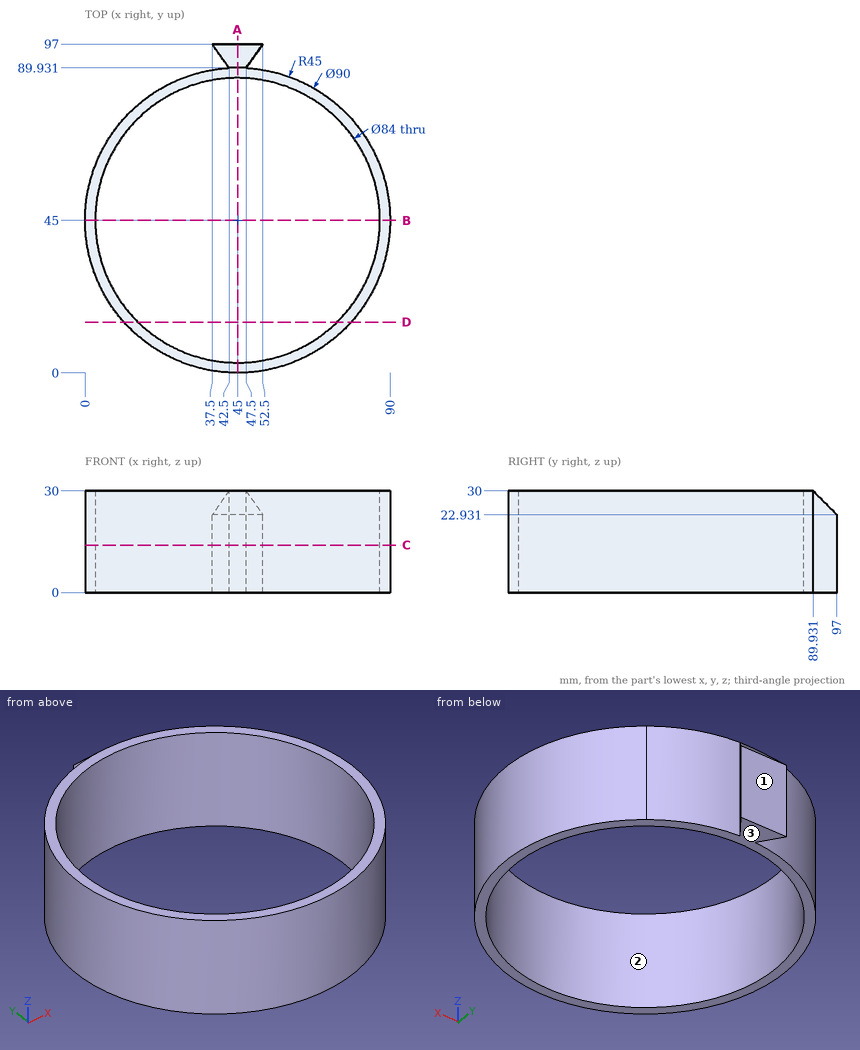
Drawing for the job (mm, zero at the part's lowest x, y, z). Round coordinates to 2 decimals unless told otherwise and drop trailing zeros. Order: outer loops, then holes, each group sorted by start corner. A loop starts at its lowest first (then second) coordinate and runs counter-clockwise, first axis right, second up. Notation, with made-up numbers: (70.25, 76) -> (124.25, 76) arc R20 ccw to (124.25, 115) -> close; hole circle Ø4 at (78, 40). An arc over 180 degrees is marked (long way). Write item = value, one per line. Start each with the question number.
(1) Pin check, flat tips, straight feed: P1, Ø12, axis at x = 11.5, z = 17, coming from the -Y side; P2, Ø2, axis at y = 38, z = 26, coming from the +X side; P3, Ø2, axis at x = 67.5, z = 26, coming from the -Y side; P4, Ø5, axis at y = 43.5, z = 12.5, coming from the -X side. Stop position of each tip, or through.
(2) Pull direction Y, two halves, no side cores. Call the marked faces 1, 2 and 3: released by +Y, released by -Y, zero draft, split by the parting line, or undercut.
(3) Cut at C-C, the plane z = 14. List the corners of the cut face in (x, y) (1 decimal).
(4) Cut at A-A, the plane x = 45. List the corners of the cut face in (y, z).
(5) Probe line 1 (Y direction, x = 45, z = 11.25); line 2 (Y direction, x = 59, z = 6.5); line 3 (X direction, y = 32, z = 15). List the from-to ranges inside material, lowest first. Write a range as [from, to].
(6) Cut at D-D, the plane y = 15. List the corners of the cut face in (x, z), then the cut area to 3 significant figures.
(7) Cut at B-B, the plane y = 45. List the corners of the cut face in (x, z).
Model answer:
q1.P1 = 9.38
q1.P2 = 89.6
q1.P3 = 5.47
q1.P4 = 0
q2.face_1 = released by +Y
q2.face_2 = undercut
q2.face_3 = zero draft
q3.outline = (37.5, 97) -> (42.5, 89.9) arc R45 ccw (long way) to (47.5, 89.9) -> (52.5, 97) -> close; hole circle Ø84 at (45, 45)
q4.outline = (0, 0) -> (3, 0) -> (3, 30) -> (0, 30) -> close; (87, 0) -> (97, 0) -> (97, 22.93) -> (89.93, 30) -> (87, 30) -> close
q5.line_1 = [0, 3], [87, 97]
q5.line_2 = [2.23, 5.4], [84.6, 87.77]
q5.line_3 = [1.92, 5.06], [84.94, 88.08]
q6.outline = (11.46, 0) -> (15.61, 0) -> (15.61, 30) -> (11.46, 30) -> close; (74.39, 0) -> (78.54, 0) -> (78.54, 30) -> (74.39, 30) -> close
q6.area = 249 mm2
q7.outline = (0, 0) -> (3, 0) -> (3, 30) -> (0, 30) -> close; (87, 0) -> (90, 0) -> (90, 30) -> (87, 30) -> close
